```python
from build123d import *

# Parameters (mm, degrees)
SKETCH1_R           = 2
SKETCH1_R_2         = 1.5
BOSS_EXTRUDE1_DEPTH = 6


with BuildPart() as part:
    # Sketch1 → Boss-Extrude1 (new body)
    with BuildSketch(Plane.XY):
        Polygon((20, 0), (60, 0), (60, -20), (60, -69.331923123), (20, -69.331923123), (20, -60), (0, -60), (0, -20), (20, -20), align=None)
        with Locations((50, -10)):
            Circle(SKETCH1_R, mode=Mode.SUBTRACT)
        with Locations((30, -10)):
            Circle(SKETCH1_R, mode=Mode.SUBTRACT)
        with Locations((10, -50)):
            Circle(SKETCH1_R, mode=Mode.SUBTRACT)
        with Locations((10, -30)):
            Circle(SKETCH1_R, mode=Mode.SUBTRACT)
        with Locations((25, -64.331923123)):
            Circle(SKETCH1_R_2, mode=Mode.SUBTRACT)
        with Locations((24.997348671, -33.331923237)):
            Circle(SKETCH1_R_2, mode=Mode.SUBTRACT)
        with Locations((56, -64.331923123)):
            Circle(SKETCH1_R_2, mode=Mode.SUBTRACT)
        with Locations((55.997348671, -33.331923123)):
            Circle(SKETCH1_R_2, mode=Mode.SUBTRACT)
    extrude(amount=BOSS_EXTRUDE1_DEPTH)


solid = part.part
```
The model under review builds one solid part; all positions refer to its coordinate system, in mm. A direction names the side the tool comes from. Round coordinates to 2 decimals unless told otherwise and drop trailing zeros. Write each loop counter-clockwise with the first axis right and the second up, starting at its lowest first coordinate (ties: lowest second). Pieces come first, ordered by that corner, then holes. Notation, with made-up numbers: (87, 58) -> (122, 58) arc R7 ccw to (122, 71) -> close; hole circle Ø6 at (70, 80.25). An arc over 180 degrees is marked (long way). Use CSV: the item, a comma, the result in double quotes.
Q1. For faces 5 (the cylindrical face through (10.923, -51.774, 2.958)), 6 (the flat face through (20, -10, 3)), 7 (the flat face through (10, -60, 3)), list the 3-axis set-ups (+Z, -Z, +X, -X, +Y, -Y) from which the entire face can be reached by the end or side of a thin tool; tool diameter is ignored.
Checks:
face 5,"+Z, -Z"
face 6,"+Z, -Z, -X, +Y"
face 7,"+Z, -Z, -X, -Y"
Q2. For pin 1 Ø1.8 at (y, z) = (-10, 2.5) entering from -X, flat-tipped, find the tip position at first contact; note if it passes through.
Checks:
pin 1,"x = 20"
Q3. Consider section A-A (x = 25). Give the boundary of the cut face in (y, z).
Checks:
outline,"(-69.33, 0) -> (-65.83, 0) -> (-65.83, 6) -> (-69.33, 6) -> close; (-62.83, 0) -> (-34.83, 0) -> (-34.83, 6) -> (-62.83, 6) -> close; (-31.83, 0) -> (0, 0) -> (0, 6) -> (-31.83, 6) -> close"
Q4. Consider section D-D (z = 1.8). State how many separate pieces and enclosed holes the cut face has, then the cut area to 3 significant figures.
Checks:
separate pieces,"1"
enclosed holes,"8"
area,"3,490 mm²"
Q5. Consider section B-B (y = -30). Give the boundary of the cut face in (x, z), then the cut area to 3 significant figures.
Checks:
outline,"(0, 0) -> (8, 0) -> (8, 6) -> (0, 6) -> close; (12, 0) -> (60, 0) -> (60, 6) -> (12, 6) -> close"
area,"336 mm²"
Q6. Consider section C-C (x = 10). Give the boundary of the cut face in (y, z).
Checks:
outline,"(-60, 0) -> (-52, 0) -> (-52, 6) -> (-60, 6) -> close; (-48, 0) -> (-32, 0) -> (-32, 6) -> (-48, 6) -> close; (-28, 0) -> (-20, 0) -> (-20, 6) -> (-28, 6) -> close"
Q7. Mouldability with a two-part tool opening along Y and no side actions: class faces 1 (the cylindrical face through (31.908, -9.399, 2.958)), 2 (the flat face through (40, -69.332, 3)), 3 (the flat face through (20, -65, 3)), 4 (the flat face through (40, 0, 3)) as released by +Y, released by -Y, zero draft, split by the parting line, or undercut.
Checks:
face 1,"undercut"
face 2,"released by -Y"
face 3,"zero draft"
face 4,"released by +Y"
Q8. To check wall thickness, follow probe 1 along Y at (x, z) = (10, 3.15); probe 2 along Y at (x, z) = (56, 4.1); probe 3 along Y at (x, z) = (18.5, 4.8). State the ranges of each line that lie inside material, in increasing order. Write a range as [from, to].
Checks:
probe 1,"[-60, -52], [-48, -32], [-28, -20]"
probe 2,"[-69.33, -65.83], [-62.83, -34.83], [-31.83, 0]"
probe 3,"[-60, -20]"
